Verification items for the finished model (mm, model axes). A direction names the side the tool comes from. Give positions to 0.01 mm unless a question says otherwise; leave off trailing zeros. Loops run counter-clockwise (first coordinate to the right, second up) from the corner with the lowest first, then second, coordinate; pieces in that order, holes last. Notation, with made-up numbers: M 51.25,59.5 L 76.25,59.5 A17 ccw 76.25,81.5 Z; hole C -30,3.5 d4. An arc over 180 degrees is marked long. Use a Markdown table: item, result.
from build123d import *

# Parameters (mm, degrees)
EXTRUDE_610_DEPTH      = 2
SKETCH_2_R             = 1.5
CUT_EXTRUDE_906_DEPTH  = 43.944731924
CUT_EXTRUDE_1170_DEPTH = 43.944731924
SKETCH_4_W             = 5
SKETCH_4_H             = 50.8
EXTRUDE_1451_DEPTH     = 8
SKETCH_5_W             = 12
SKETCH_5_H             = 6
CAN_DEPTH              = 7
PATTERN_LINEAR_1_COUNT = 2
PATTERN_LINEAR_1_PITCH = 10
SKETCH_6_W             = 4
SKETCH_6_H             = 10
EXTRUDE_2243_DEPTH     = 8
SKETCH_7_W             = 13
SKETCH_7_H             = 19
EXTRUDE_2697_DEPTH     = 5
SKETCH_8_W             = 6.5
SKETCH_8_H             = 6.5
EXTRUDE_2917_DEPTH     = 3
SKETCH_9_W             = 3
SKETCH_9_H             = 8
UART_DEPTH             = 8
EXTRUDE_3952_DEPTH     = 4
FILLET_1_R             = 3.5


with BuildPart() as part:
    # Эскиз1 → Extrude 610 (new body)
    with BuildSketch(Plane(origin=(0, 0, 0), x_dir=(1, 0, 0), z_dir=(0, 1, 0))):
        Polygon((-28, 32.5), (28, 32.5), (28, -32.5), (9, -32.5), (9, -27.5), (-9, -27.5), (-9, -32.5), (-28, -32.5), align=None)
    extrude(amount=EXTRUDE_610_DEPTH)

    # Эскиз2 → Cut-Extrude 906 (cut, through all)
    with BuildSketch(Plane(origin=(0, 2, 0), x_dir=(1, 0, 0), z_dir=(0, 1, 0))):
        with Locations(Location((-24.5, 29, 0), (0, 0, 270))):
            Circle(SKETCH_2_R)
        with Locations(Location((24.5, 29, 0), (0, 0, 270))):
            Circle(SKETCH_2_R)
        with Locations(Location((24.5, -29, 0), (0, 0, 270))):
            Circle(SKETCH_2_R)
    extrude(amount=-CUT_EXTRUDE_906_DEPTH, mode=Mode.SUBTRACT)

    # Эскиз3 → Cut-Extrude 1170 (cut, through all)
    with BuildSketch(Plane(origin=(0, 2, 0), x_dir=(1, 0, 0), z_dir=(0, 1, 0))):
        with BuildLine():
            Line((7.5, 13), (24.5, 13))
            ThreePointArc((24.5, 13), (25.5, 12), (24.5, 11))
            Line((24.5, 11), (7.5, 11))
            ThreePointArc((7.5, 11), (6.5, 12), (7.5, 13))
        make_face()
    extrude(amount=-CUT_EXTRUDE_1170_DEPTH, mode=Mode.SUBTRACT)

    # Эскиз4 → Extrude 1451 (add)
    with BuildSketch(Plane.XZ):
        with Locations((-24.5, 0)):
            Rectangle(SKETCH_4_W, SKETCH_4_H)
    extrude(amount=EXTRUDE_1451_DEPTH)

    # Эскиз5 → CAN разъем (add)
    with BuildSketch(Plane(origin=(0, 2, 0), x_dir=(1, 0, 0), z_dir=(0, 1, 0))):
        with Locations((0, -22.5)):
            Rectangle(SKETCH_5_W, SKETCH_5_H)
    can = extrude(amount=CAN_DEPTH)

    # Линейный массив1: CAN разъем ×2
    with Locations(*[(0, 0, -i * PATTERN_LINEAR_1_PITCH) for i in range(1, PATTERN_LINEAR_1_COUNT)]):
        add(can)

    # Эскиз6 → Extrude 2243 (add)
    with BuildSketch(Plane(origin=(0, 2, 0), x_dir=(1, 0, 0), z_dir=(0, 1, 0))):
        with Locations((-10, -17.5)):
            Rectangle(SKETCH_6_W, SKETCH_6_H)
    extrude(amount=EXTRUDE_2243_DEPTH)

    # Эскиз7 → Extrude 2697 (add)
    with BuildSketch(Plane(origin=(0, 2, 0), x_dir=(1, 0, 0), z_dir=(0, 1, 0))):
        with Locations((17.5, -9)):
            Rectangle(SKETCH_7_W, SKETCH_7_H)
    extrude(amount=EXTRUDE_2697_DEPTH)

    # Эскиз8 → Extrude 2917 (add)
    with BuildSketch(Plane(origin=(0, 7, 0), x_dir=(1, 0, 0), z_dir=(0, 1, 0))):
        with Locations((17.5, -4.75)):
            Rectangle(SKETCH_8_W, SKETCH_8_H)
    extrude(amount=EXTRUDE_2917_DEPTH)

    # Эскиз9 → uart (add)
    with BuildSketch(Plane(origin=(0, 2, 0), x_dir=(1, 0, 0), z_dir=(0, 1, 0))):
        with Locations((-17.5, -9.5)):
            Rectangle(SKETCH_9_W, SKETCH_9_H)
    extrude(amount=UART_DEPTH)

    # Эскиз10 → Extrude 3952 (add)
    with BuildSketch(Plane(origin=(0, 2, 0), x_dir=(1, 0, 0), z_dir=(0, 1, 0))):
        with BuildLine():
            Line((3.75, -0.25), (3.75, 6.25))
            ThreePointArc((3.75, 6.25), (5.5, 8), (7.25, 6.25))
            Line((7.25, 6.25), (7.25, -0.25))
            ThreePointArc((7.25, -0.25), (5.5, -2), (3.75, -0.25))
        make_face()
    extrude(amount=EXTRUDE_3952_DEPTH)

    # Скругление1
    fillet_1_edges = [part.edges().sort_by_distance(p)[0] for p in [
        (-28, 1, -32.5),
        (28, 1, -32.5),
        (28, 1, 32.5),
        (9, 1, 27.5),
        (-9, 1, 27.5),
        (-28, 1, 32.5),
    ]]
    fillet(fillet_1_edges, radius=FILLET_1_R)


solid = part.part
(1) Cross-section at C-C on z = -2. Record the cut outline in (x, y).
Results below:
| item | result |
|---|---|
| outline | M -28,0 L -27,0 L -27,-8 L -22,-8 L -22,0 L 28,0 L 28,2 L 7.25,2 L 7.25,6 L 3.75,6 L 3.75,2 L -28,2 Z |
(2) Draft check along X on faces 1 (the flat face through (-27, -4, 0)), 2 (the flat face through (0, 0, 0)), 3 (the flat face through (-16, 6, 10)). Enter one of: +X half, -X half, draft (parallel to the pull), parting line (faces both ways), or undercut.
Results below:
| item | result |
|---|---|
| face 1 | -X half |
| face 2 | draft |
| face 3 | undercut |
(3) Cross-section at D-D on y = -5. Record the cut outline in (x, z).
Results below:
| item | result |
|---|---|
| outline | M -27,-25.4 L -22,-25.4 L -22,25.4 L -27,25.4 Z |
(4) Material ranges on line 1 (X direction, y = 0.95, z = -29); line 2 (Z direction, x = 19, y = 0.5); line 3 (X direction, y = -3.5, z = -7), recorded low to high.
Results below:
| item | result |
|---|---|
| line 1 | -28 to -26, -23 to 23, 26 to 28 |
| line 2 | -32.5 to -13, -11 to 32.5 |
| line 3 | -27 to -22 |
(5) Gauge pin test, flat ends, axial feed: P1, Ø5.5, axis at x = -2, y = 7, coming from the -Z side; P2, Ø6.5, axis at y = 6.5, z = 15, coming from the -X side; P3, Ø5.5, axis at x = 1.5, y = 4, coming from the +Z side. Record the tip position at first contact, or that the pin passes through.
Results below:
| item | result |
|---|---|
| P1 | z = 9.5 |
| P2 | x = -19 |
| P3 | z = 27.5 |
(6) Cross-section at B-B on x = 2. Record the cut outline in (y, z), then the cut area to 3 significant figures.
Results below:
| item | result |
|---|---|
| outline | M 0,-32.5 L 2,-32.5 L 2,9.5 L 9,9.5 L 9,15.5 L 2,15.5 L 2,19.5 L 9,19.5 L 9,25.5 L 2,25.5 L 2,27.5 L 0,27.5 Z |
| area | 204 mm^2 |
(7) Cross-section at A-A on y = 3. Record the cut outline in (x, z), then the cut area to 3 significant figures.
Results below:
| item | result |
|---|---|
| outline | M -19,5.5 L -16,5.5 L -16,13.5 L -19,13.5 Z; M -12,12.5 L -8,12.5 L -8,22.5 L -12,22.5 Z; M -6,9.5 L 6,9.5 L 6,15.5 L -6,15.5 Z; M -6,19.5 L 6,19.5 L 6,25.5 L -6,25.5 Z; M 3.75,-6.25 A1.75 ccw 7.25,-6.25 L 7.25,0.25 A1.75 ccw 3.75,0.25 Z; M 11,-0.5 L 24,-0.5 L 24,18.5 L 11,18.5 Z |
| area | 487 mm^2 |
(8) Set-up check for faces 4 (the flat face through (6, 6, -3)), 5 (the flat face through (9, 1, 32)), 6 (the flat face through (-10, 6, 22.5)): record each of +Z, -Z, +X, -X, +Y, -Y from which the full face is reachable in a straight line by a thin tool's end or side.
Results below:
| item | result |
|---|---|
| face 4 | -Z, -X, +Y |
| face 5 | +Z, +Y, -Y |
| face 6 | +Z, -X, +Y |
